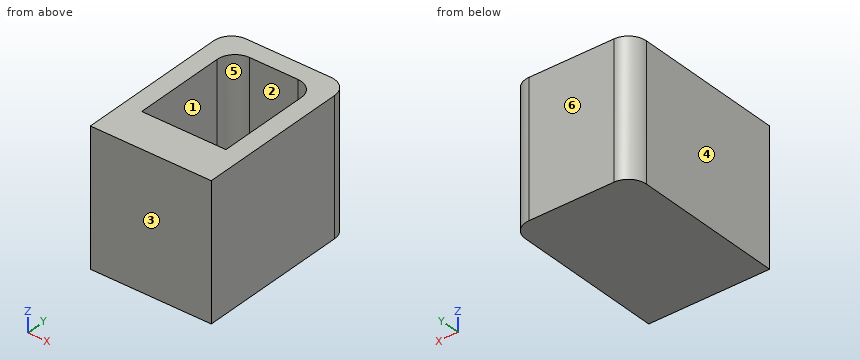
Autodesk Inventor part; units mm, degrees
ref_plane "YZ Plane" through (0, 0, 0) normal (1, 0, 0) x (0, 1, 0)
ref_plane "XZ Plane" through (0, 0, 0) normal (0, 1, 0) x (-1, 0, 0)
ref_plane "XY Plane" through (0, 0, 0) normal (0, 0, 1) x (1, 0, 0)
sketch "Sketch1" plane through (0, 0, 0) normal (0, 0, 1) x (1, 0, 0)
  line L0 (0, 0) -> (-13.5, 0)
  line L1 (-13.5, 0) -> (-13.5, 19)
  line L2 (-13.5, 19) -> (0, 19)
  line L3 (0, 19) -> (0, 0)
  dimension "d0" = 13.5
  dimension "d1" = 19
extrude "Extrusion1" add sketch "Sketch1" along normal blind 10 and the other way blind 5
sketch "Sketch2" plane through (0, 0, 10) normal (0, 0, 1) x (1, 0, 0)
  line L0 (-13.5, 19) -> (-13.5, 0)
  line L1 (-13.5, 0) -> (-11.45, 0)
  line L2 (-11.45, 0) -> (-11.45, 4.55)
  line L3 (-11.45, 4.55) -> (-13.5, 4.55)
  line L4 (-13.5, 4.55) -> (-13.5, 0)
  line L5 (0, 19) -> (-13.5, 19)
  line L6 (0, 19) -> (-2.05, 19)
  line L7 (-2.05, 19) -> (-2.05, 16.95)
  line L8 (-2.05, 16.95) -> (0, 16.95)
  line L9 (0, 16.95) -> (0, 19)
  line L10 (-11.45, 4.55) -> (-2.05, 4.55)
  line L11 (-2.05, 4.55) -> (-2.05, 16.95)
  line L12 (-2.05, 16.95) -> (-11.45, 16.95)
  line L13 (-11.45, 16.95) -> (-11.45, 4.55)
  point P0 (0, 0)
  dimension "d4" = 2.05
  dimension "d5" = 4.55
  dimension "d6" = 2.05
  dimension "d7" = 2.05
extrude "Extrusion2" cut sketch "Sketch2" against normal blind 10 contours L13 L12 L11 L10
fillet "Fillet1" radius 2 2 edges at (-11.45, 16.95, 5) (-2.05, 16.95, 5)
fillet "Fillet9" radius 2 2 edges at (0, 19, 2.5) (-13.5, 19, 2.5)
properties part number "Rod"
Design review of the part built by this model. Coordinates are the model's own, in mm. Face numbers are marked on the shaded views. A direction names the side the tool comes from. Coordinates: 2 decimals unless noted, no trailing zeros. Loops run counter-clockwise (first coordinate to the right, second up) from the corner with the lowest first, then second, coordinate; pieces in that order, holes last. Notation, with made-up numbers: M -30.75,12 L -22.75,12 A23 cw -22.75,43 Z; hole C 57.5,39.25 d9. An arc over 180 degrees is marked long. Use one line per item in the form item = value.
(1) Consider section C-C (y = 9). Write out the cut boundary in (x, z).
Return value:
outline = M -13.5,-5 L 0,-5 L 0,10 L -2.05,10 L -2.05,0 L -11.45,0 L -11.45,10 L -13.5,10 Z
(2) Consider section B-B (x = -8.5). Write out the cut boundary in (y, z), and give its area (3 significant figures).
Return value:
outline = M 0,-5 L 19,-5 L 19,10 L 16.95,10 L 16.95,0 L 4.55,0 L 4.55,10 L 0,10 Z
area = 161 mm2
(3) For line 1 along X through (y, z) = (14.5, 5); line 2 along Y through (x, z) = (-6.5, 3.25); line 3 along Z through (x, y) = (-10.5, 6.25), list the stretches that pass through material, from the lowest coordinate up. Write a range as from..to.
Return value:
line_1 = -13.5..-11.45, -2.05..0
line_2 = 0..4.55, 16.95..19
line_3 = -5..0
(4) For the marked faces 5 and 6, list the 3-axis set-ups (+Z, -Z, +X, -X, +Y, -Y) from which the entire face can be reached by the end or side of a thin tool; tool diameter is ignored.
Return value:
face_5 = +Z
face_6 = +Z, -Z, +X, -X, +Y
(5) Consider section A-A (z = 2.5). Write out the cut boundary in (x, y).
Return value:
outline = M -13.5,0 L 0,0 L 0,17 A2 ccw -2,19 L -11.5,19 A2 ccw -13.5,17 Z; hole M -11.45,4.55 L -2.05,4.55 L -2.05,14.95 A2 ccw -4.05,16.95 L -9.45,16.95 A2 ccw -11.45,14.95 Z
(6) Clearance check with flat-ended pins moving along their axes: P1, Ø3, axis at x = -9, y = 14.5, coming from the +Z side; P2, Ø6, axis at y = 4.5, z = 7.5, coming from the +X side. State where each tip first meets the part, or that it passes through.
Return value:
P1 = 0
P2 = 0
(7) Draft analysis for pull direction Y (two halves, no side actions). For the marked faces 1, 2, 3 and 4, state which applies: pulls with the +Y half, pulls with the -Y half, needs draft (parallel to the pull), parting line crosses it, or undercut.
Return value:
face_1 = undercut
face_2 = undercut
face_3 = pulls with the -Y half
face_4 = needs draft
